Input: dimensioned drawing with shaded views. Units: mm. Origin: part minimum x, y, z. Give positions to 0.01 mm unless a question says otherwise; leave off trailing zeros. Write each loop counter-clockwise with the first axis right and the second up, starting at its lowest first coordinate (ties: lowest second). Pieces come first, ordered by that corner, then holes. Notation, with made-up numbers: (40, 76) - (78, 76) arc R22 cw to (78, 112) - close; hole circle Ø1 at (68, -40). An arc over 180 degrees is marked (long way). Answer as a JSON object with one key per item and string values. Group by question number.
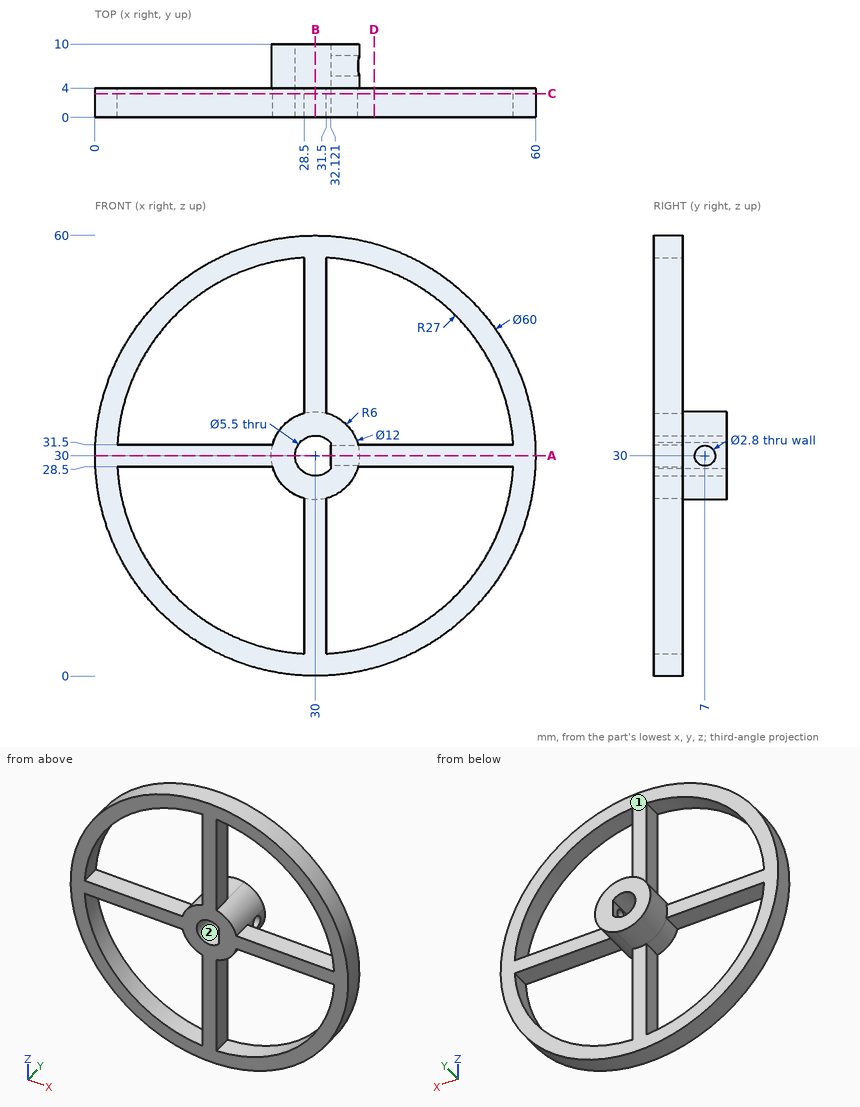
1) Line query: line 1 along X through (y, z) = (1.5, 25) (1 decimal); line 2 along Y through (x, z) = (35, 30); line 3 along X through (y, z) = (3.5, 22). Output: solid intervals per line, ascending. Write a range as from..to.
2) Cut plane C-C on y = 3.25. Return the cut outline in (x, z).
3) Pin query (flat end, axial travel): P1, Ø4, axis at x = 19, y = 4.5, coming from the -Z side; P2, Ø2, axis at x = 36.5, y = 3.5, coming from the +Z side; P3, Ø1.2, axis at y = 3, z = 9.5, coming from the +X side. Return the tip coordinate at first contact, or that it passes through.
4) Cut plane A-A on z = 30. Return the cut outline in (x, y).
5) Mould query, pull axis X, two halves, no side actions, for the marked faces 1 and 2. Classes: +X half, -X half, draft (parallel to the pull), parting line (faces both ways), or undercut.
6) Cut plane B-B on x = 30. Return the cut outline in (y, z), and give its area (3 significant figures).
7) Cut plane D-D on x = 38. Return the cut outline in (y, z), and give its area (3 significant figures).
Filled in:
{
 "1": {"line 1": "x = 0.4..3.5, 26.7..33.3, 56.5..59.6", "line 2": "y = 0..5.6, 8.4..10", "line 3": "x = 1.09..4.21, 28.5..31.5, 55.79..58.91"},
 "2": {"outline": "circle Ø60 at (30, 30); hole (3.04, 28.5) arc R27 ccw to (28.5, 3.04) - (28.5, 24.19) arc R6 cw to (24.19, 28.5) - close; hole (3.04, 31.5) - (24.19, 31.5) arc R6 cw to (28.5, 35.81) - (28.5, 56.96) arc R27 ccw to start; hole (31.5, 3.04) arc R27 ccw to (56.96, 28.5) - (35.81, 28.5) arc R6 cw to (31.5, 24.19) - close; hole (31.5, 35.81) arc R6 cw to (35.81, 31.5) - (56.96, 31.5) arc R27 ccw to (31.5, 56.96) - close; hole (32.12, 28.25) - (32.12, 31.75) arc R2.75 ccw (long way) to start"},
 "3": {"P1": "stops at z = 1.4", "P2": "stops at z = 59.49", "P3": "stops at x = 52.45"},
 "4": {"outline": "(0, 0) - (27.25, 0) - (27.25, 10) - (24, 10) - (24, 4) - (0, 4) - close; (32.12, 0) - (60, 0) - (60, 4) - (36, 4) - (36, 5.6) - (32.12, 5.6) - close; (32.12, 8.4) - (36, 8.4) - (36, 10) - (32.12, 10) - close"},
 "5": {"face 1": "draft", "face 2": "undercut"},
 "6": {"outline": "(0, 0) - (4, 0) - (4, 24) - (10, 24) - (10, 27.25) - (0, 27.25) - close; (0, 32.75) - (10, 32.75) - (10, 36) - (4, 36) - (4, 60) - (0, 60) - close", "area": "257 mm²"},
 "7": {"outline": "(0, 1.09) - (4, 1.09) - (4, 4.21) - (0, 4.21) - close; (0, 28.5) - (4, 28.5) - (4, 31.5) - (0, 31.5) - close; (0, 55.79) - (4, 55.79) - (4, 58.91) - (0, 58.91) - close", "area": "37.0 mm²"}
}
